from build123d import *

# Parameters (mm, degrees)
SKETCH_1_W          = 134
SKETCH_1_H          = 33
EXTRUDE_1_DEPTH     = 40
EXTRUDE_START       = 19
SKETCH_2_W          = 134
SKETCH_2_H          = 33
EXTRUDE_2_DEPTH     = 3
SKETCH_3_W          = 4.5
SKETCH_3_H          = 12
CUT_EXTRUDE_1_DEPTH = 79.625695545
SKETCH_4_W          = 134
SKETCH_4_H          = 55
CUT_EXTRUDE_2_DEPTH = 20
SKETCH_6_W          = 14
SKETCH_6_H          = 7
CUT_EXTRUDE_3_DEPTH = 10
SKETCH_7_W          = 8
SKETCH_7_H          = 14
CUT_EXTRUDE_4_DEPTH = 10
SKETCH_8_W          = 133
SKETCH_8_H          = 3
CUT_EXTRUDE_5_DEPTH = 10


with BuildPart() as part:
    # 草图1 → 凸台-拉伸1 (new body)
    with BuildSketch(Plane.XY):
        with BuildLine():
            Line((-64, 29), (64, 29))
            ThreePointArc((64, 29), (68.242640687, 27.242640687), (70, 23))
            Line((70, 23), (70, -23))
            ThreePointArc((70, -23), (68.242640687, -27.242640687), (64, -29))
            Line((64, -29), (-64, -29))
            ThreePointArc((-64, -29), (-68.242640687, -27.242640687), (-70, -23))
            Line((-70, -23), (-70, 23))
            ThreePointArc((-70, 23), (-68.242640687, 27.242640687), (-64, 29))
        make_face()
        Rectangle(SKETCH_1_W, SKETCH_1_H, mode=Mode.SUBTRACT)
    extrude(amount=EXTRUDE_1_DEPTH)

    # 草图2 → 凸台-拉伸2 (add)
    with BuildSketch(Plane.XY.offset(EXTRUDE_START)):
        Rectangle(SKETCH_2_W, SKETCH_2_H)
    extrude(amount=EXTRUDE_2_DEPTH)

    # 草图3 → 切除-拉伸1 (cut, through all)
    with BuildSketch(Plane(origin=(0, 0, 19), x_dir=(-1, 0, 0), z_dir=(0, 0, -1))):
        with Locations((64.75, -0.409735633)):
            Rectangle(SKETCH_3_W, SKETCH_3_H)
    extrude(amount=-CUT_EXTRUDE_1_DEPTH, mode=Mode.SUBTRACT)

    # 草图4 → 切除-拉伸2 (cut)
    with BuildSketch(Plane.XY.offset(40)):
        Rectangle(SKETCH_4_W, SKETCH_4_H)
    extrude(amount=-CUT_EXTRUDE_2_DEPTH, mode=Mode.SUBTRACT)

    # 草图6 → 切除-拉伸3 (cut)
    with BuildSketch(Plane(origin=(0, 29, 0), x_dir=(1, 0, 0), z_dir=(0, 1, 0))):
        with Locations((0, -33.5)):
            Rectangle(SKETCH_6_W, SKETCH_6_H)
    extrude(amount=-CUT_EXTRUDE_3_DEPTH, mode=Mode.SUBTRACT)

    # 草图7 → 切除-拉伸4 (cut)
    with BuildSketch(Plane.ZY.offset(-67)):
        with Locations((25, -6.5)):
            Rectangle(SKETCH_7_W, SKETCH_7_H)
    extrude(amount=-CUT_EXTRUDE_4_DEPTH, mode=Mode.SUBTRACT)

    # 草图8 → 切除-拉伸5 (cut)
    with BuildSketch(Plane(origin=(0, 0, 0), x_dir=(-1, 0, 0), z_dir=(0, 0, -1))):
        with Locations((0.239080463, 24)):
            Rectangle(SKETCH_8_W, SKETCH_8_H)
        with Locations((0.239080463, -24)):
            Rectangle(SKETCH_8_W, SKETCH_8_H)
    extrude(amount=-CUT_EXTRUDE_5_DEPTH, mode=Mode.SUBTRACT)


solid = part.part
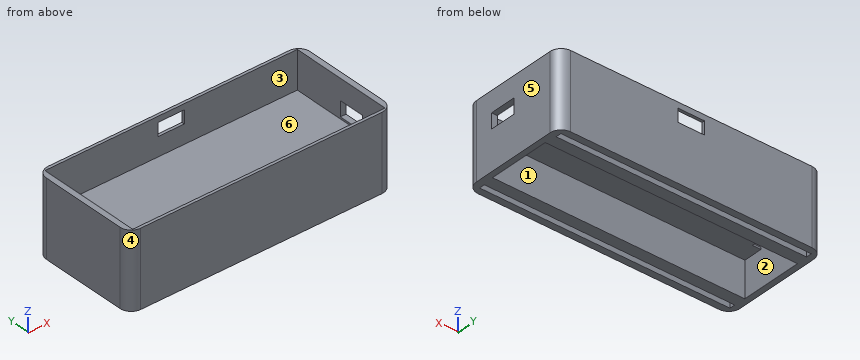
Geometry: final body of the model. Coordinates: model frame, mm. Face numbers are marked on the shaded views. A direction names the side the tool comes from. Give positions to 0.01 mm unless a question says otherwise; leave off trailing zeros. Loops run counter-clockwise (first coordinate to the right, second up) from the corner with the lowest first, then second, coordinate; pieces in that order, holes last. Notation, with made-up numbers: (27, -12.5) - (51, -12.5) arc R23 ccw to (51, 7.5) - close; hole circle Ø2 at (37, 11). An arc over 180 degrees is marked (long way). One line per question, with ' | ' between items. Start each with the question number.
(1) Pull-direction query (Y, two-part tool) for the marked faces 4, 5 and 6; classes: released by +Y, released by -Y, zero draft, split by the parting line, or undercut.
(2) Reachability of the marked faces 1, 2 and 3 from +Z, -Z, +X, -X, +Y, -Y: full face, straight path, thin tool, end or side. Return the list, or none.
(3) Contact query for flat-ended pins moving along their axis: pin 1 (4 mm diameter, centred on x = 22, y = -8, fed in from -Z); pin 2 (0.8 mm diameter, centred on x = -65, z = 19.5, fed in from -Y); pin 3 (1.5 mm diameter, centred on y = 24, z = 4, fed in from +X). Output: stop coordinate, or through.
(4) Section query C-C on x = -48.5. Return loops of the section in (y, z).
(5) Ray query, line 1 (Y direction, x = -63, z = 7.5); line 2 (X direction, y = 14.5, z = 23.5); line 3 (Y direction, x = 10, z = 10.5). Return the intervals inside material, ascending. Write a range as from..to.
(6) Section query B-B on z = 11.5. Return loops of the section in (x, y).
(7) Section query D-D on z = 26.5. Return loops of the section in (x, y), then the cut area to 3 significant figures.
(8) Section query A-A on y = 2.5. Return loops of the section in (x, z).
The answers:
1) face 4: released by -Y | face 5: zero draft | face 6: undercut
2) face 1: -Z | face 2: none | face 3: +Z
3) pin 1: z = 19 | pin 2: y = -28.97 | pin 3: x = 69.99
4) outline: (-29, 0) - (-25.5, 0) - (-25.5, 10) - (-22.5, 10) - (-22.5, 0) - (-16.5, 0) - (-16.5, 19) - (16.5, 19) - (16.5, 0) - (22.5, 0) - (22.5, 10) - (25.5, 10) - (25.5, 0) - (29, 0) - (29, 40) - (27.5, 40) - (27.5, 20) - (-27.5, 20) - (-27.5, 40) - (-29, 40) - close
5) line 1: -29..-25.5, -22.5..-16.5, 16.5..22.5, 25.5..29 | line 2: -70..-67, 67..70 | line 3: -29..-16.5, 16.5..29
6) outline: (-70, -23) arc R6 ccw to (-64, -29) - (64, -29) arc R6 ccw to (70, -23) - (70, 23) arc R6 ccw to (64, 29) - (-64, 29) arc R6 ccw to (-70, 23) - close; hole (-67, -16.5) - (67, -16.5) - (67, 16.5) - (-67, 16.5) - close
7) outline: (-70, -23) arc R6 ccw to (-64, -29) - (64, -29) arc R6 ccw to (70, -23) - (70, -13.5) - (67, -13.5) - (67, -27.5) - (-67, -27.5) - (-67, 27.5) - (67, 27.5) - (67, 0.5) - (70, 0.5) - (70, 23) arc R6 ccw to (64, 29) - (-64, 29) arc R6 ccw to (-70, 23) - close | area: 677 mm2
8) outline: (-70, 0) - (-67, 0) - (-67, 40) - (-70, 40) - close; (-62.5, 19) - (67, 19) - (67, 0) - (70, 0) - (70, 40) - (67, 40) - (67, 20) - (-62.5, 20) - close
